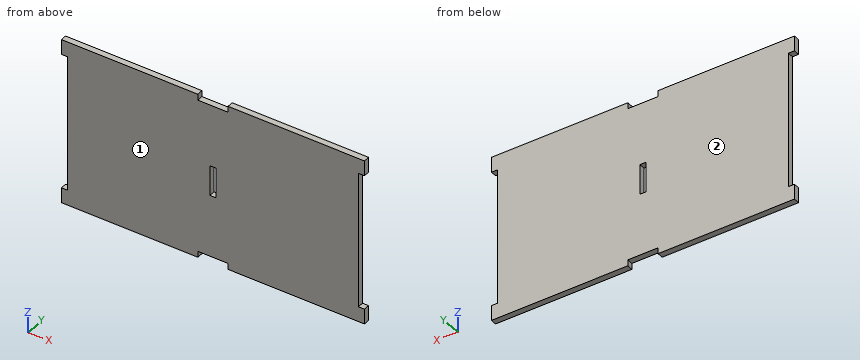
from build123d import *

# Parameters (mm, degrees)
SKETCH1_W           = 2
SKETCH1_H           = 10
BOSS_EXTRUDE1_DEPTH = 2


with BuildPart() as part:
    # Sketch1 → Boss-Extrude1 (new body)
    with BuildSketch(Plane(origin=(0, 0, 0), x_dir=(1, 0, 0), z_dir=(0, 1, 0))):
        Polygon((-50, 22.5), (-48, 22.5), (-48, -22.5), (-50, -22.5), (-50, -27.5), (-5, -27.5), (-5, -25.5), (5, -25.5), (5, -27.5), (50, -27.5), (50, -22.5), (48, -22.5), (48, 22.5), (50, 22.5), (50, 27.5), (5, 27.5), (5, 25.5), (-5, 25.5), (-5, 27.5), (-50, 27.5), align=None)
        Rectangle(SKETCH1_W, SKETCH1_H, mode=Mode.SUBTRACT)
    extrude(amount=BOSS_EXTRUDE1_DEPTH)


solid = part.part
Could you check a few things on this model? Use its own coordinates, in mm. Face numbers are marked on the shaded views. Give positions to 0.01 mm unless a question says otherwise; leave off trailing zeros. Order: outer loops, then holes, each group sorted by start corner. A loop starts at its lowest first (then second) coordinate and runs counter-clockwise, first axis right, second up.
1. I need wall thicknesses on L1, parallel to X at y = 1.2, z = 1; L2, parallel to X at y = 0.65, z = 21.5. Which ranges of each line are inside material? Lowest first, please.
Answers below:
L1: x = -48 to -1, 1 to 48
L2: x = -48 to 48
2. Suppose I cut it at B-B (y = 1.35). Write out the boundary of the cut face in (x, z), plus the area to 3 significant figures.
Answers below:
outline: (-50, -27.5) - (-5, -27.5) - (-5, -25.5) - (5, -25.5) - (5, -27.5) - (50, -27.5) - (50, -22.5) - (48, -22.5) - (48, 22.5) - (50, 22.5) - (50, 27.5) - (5, 27.5) - (5, 25.5) - (-5, 25.5) - (-5, 27.5) - (-50, 27.5) - (-50, 22.5) - (-48, 22.5) - (-48, -22.5) - (-50, -22.5) - close; hole (-1, -5) - (1, -5) - (1, 5) - (-1, 5) - close
area: 5,260 mm2
3. Thinking about a two-plate mould opening in Y: for the marked faces 1 and 2, which applies, +Y half, -Y half, draft (parallel to the pull), parting line (faces both ways), or undercut?
Answers below:
face 1: -Y half
face 2: +Y half
4. For pin 1 (0.6 mm diameter, centred on x = 1, y = 0.5, fed in from -Z); pin 2 (1 mm diameter, centred on x = -1.5, y = 1, fed in from +Z); pin 3 (1 mm diameter, centred on y = 0.5, z = -20.5, fed in from +X), each with a flat end and sliding along its axis, tell me the tip position at first contact or that it passes through.
Answers below:
pin 1: stops at z = -25.5
pin 2: stops at z = 25.5
pin 3: stops at x = 48
5. Suppose I cut it at A-A (z = 1). Write out the boundary of the cut face in (x, y), plus the area to 3 significant figures.
Answers below:
outline: (-48, 0) - (-1, 0) - (-1, 2) - (-48, 2) - close; (1, 0) - (48, 0) - (48, 2) - (1, 2) - close
area: 188 mm2
6. Suppose I cut it at C-C (z = -8.5). Write out the boundary of the cut face in (x, y).
Answers below:
outline: (-48, 0) - (48, 0) - (48, 2) - (-48, 2) - close
